```python
from build123d import *

# Parameters (mm, degrees)
BOSS_EXTRUDE1_DEPTH = 181.2
CUT_EXTRUDE1_DEPTH  = 11.4


with BuildPart() as part:
    # Sketch1 → Boss-Extrude1 (new body, symmetric)
    with BuildSketch(Plane(origin=(0, 0, 0), x_dir=(0, 0, -1), z_dir=(1, 0, 0))):
        Polygon((-4, 5), (-4, 0), (4, 0), (4, 5), (5.2, 5), (5.2, -1.2), (-5.2, -1.2), (-5.2, 5), align=None)
    extrude(amount=BOSS_EXTRUDE1_DEPTH, both=True)

    # Sketch3 → Cut-Extrude1 (cut, through all)
    with BuildSketch(Plane.XY.offset(5.2)):
        Polygon((-181.2, 5), (-181.2, -1.2), (-175, 5), align=None)
        Polygon((181.2, 5), (181.2, -1.2), (175, 5), align=None)
    extrude(amount=-CUT_EXTRUDE1_DEPTH, mode=Mode.SUBTRACT)


solid = part.part
```
Build history of the part. All positions in model axes, mm. Round coordinates to 2 decimals unless told otherwise and drop trailing zeros. Write each loop counter-clockwise with the first axis right and the second up, starting at its lowest first coordinate (ties: lowest second). Pieces come first, ordered by that corner, then holes. Notation, with made-up numbers: (-21.5, -34) - (26.5, -34) arc R15 cw to (26.5, -14) - close; hole circle Ø4 at (-24, 65). An arc over 180 degrees is marked (long way). Answer as CSV lines item,"result".
Q1. Drill centre lines: probe 1 along Z at (x, y) = (117, 4.75); probe 2 along Y at (x, z) = (-44, 3.25); probe 3 along X at (y, z) = (4.25, 4.25). Where is each one in solid material? Low to high. Write a range as [from, to].
Report:
probe 1,"z = [-5.2, -4], [4, 5.2]"
probe 2,"y = [-1.2, 0]"
probe 3,"x = [-175.75, 175.75]"
Q2. Cut at C-C (z = -2.25). Write the cut outline in (x, y), and give its area (3 significant figures).
Report:
outline,"(-181.2, -1.2) - (181.2, -1.2) - (180, 0) - (-180, 0) - close"
area,"433 mm^2"
Q3. Cut at B-B (x = 21.5). Write the cut outline in (y, z), and give its area (3 significant figures).
Report:
outline,"(-1.2, -5.2) - (5, -5.2) - (5, -4) - (0, -4) - (0, 4) - (5, 4) - (5, 5.2) - (-1.2, 5.2) - close"
area,"24.5 mm^2"
Q4. Drop a flat-ended pin along its axis: pin 1 (2.5 mm diameter, centred on x = 44.5, z = 2, fed in from +Y). Give the stop position or say it passes through.
Report:
pin 1,"stops at y = 0"
Q5. Cut at A-A (y = 2.75). Write the cut outline in (x, z).
Report:
outline,"(-177.25, -5.2) - (177.25, -5.2) - (177.25, -4) - (-177.25, -4) - close; (-177.25, 4) - (177.25, 4) - (177.25, 5.2) - (-177.25, 5.2) - close"
Q6. Pull direction Z, two halves, no side cores. Call faces 1 (the flat face through (3, 0, 0)), 2 (the flat face through (3, 2, 5.2)), 3 (the flat face through (-180.2, -0.2, 0.1)): +Z half, -Z half, draft (parallel to the pull), parting line (faces both ways), or undercut.
Report:
face 1,"undercut"
face 2,"+Z half"
face 3,"draft"
